Geometry: final body of the model. Coordinates: model frame, mm. Face numbers are marked on the shaded views. Give positions to 0.01 mm unless a question says otherwise; leave off trailing zeros. Loops run counter-clockwise (first coordinate to the right, second up) from the corner with the lowest first, then second, coordinate; pieces in that order, holes last. Notation, with made-up numbers: (10, 40) - (27, 40) arc R23 cw to (27, 76) - close; hole circle Ø9 at (63, 48.25). An arc over 180 degrees is marked (long way). Use one line per item in the form item = value.
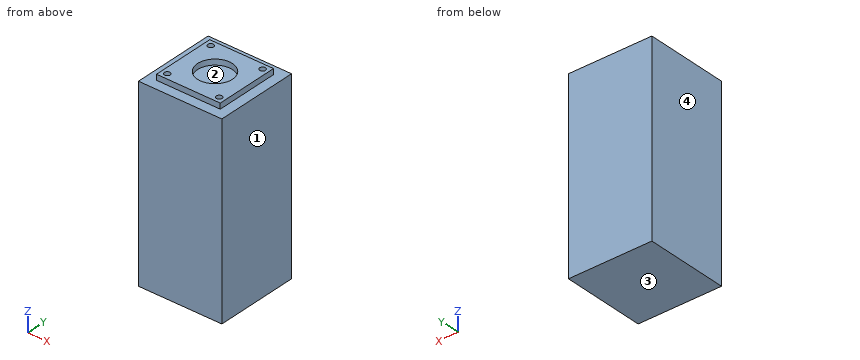
Autodesk Inventor part; units mm, degrees
ref_plane "YZ Plane" through (0, 0, 0) normal (1, 0, 0) x (0, 1, 0)
ref_plane "XZ Plane" through (0, 0, 0) normal (0, 1, 0) x (-1, 0, 0)
ref_plane "XY Plane" through (0, 0, 0) normal (0, 0, 1) x (1, 0, 0)
sketch "Sketch1" plane through (0, 0, 0) normal (0, 0, 1) x (1, 0, 0)
  line L0 (-11.25, 11.25) -> (11.25, 11.25)
  line L1 (11.25, 11.25) -> (11.25, -11.25)
  line L2 (11.25, -11.25) -> (-11.25, -11.25)
  line L3 (-11.25, -11.25) -> (-11.25, 11.25)
  line L4 (-11.25, 11.25) -> (11.25, -11.25) construction
  line L5 (11.25, 11.25) -> (-11.25, -11.25) construction
  point P0 (0, 0)
  dimension "d0" = 22.5
  dimension "d1" = 22.5
extrude "Extrusion1" add sketch "Sketch1" along normal mid plane 50.5
sketch "Sketch8" plane through (0, 0, 25.25) normal (0, 0, 1) x (1, 0, 0)
  line L0 (-8.6, 8.6) -> (8.6, 8.6)
  line L1 (8.6, 8.6) -> (8.6, -8.6)
  line L2 (8.6, -8.6) -> (-8.6, -8.6)
  line L3 (-8.6, -8.6) -> (-8.6, 8.6)
  line L4 (-8.6, 8.6) -> (8.6, -8.6) construction
  line L5 (8.6, 8.6) -> (-8.6, -8.6) construction
  circle A0 centre (0, 0) radius 4.715
  dimension "d41" = 17.2
  dimension "d42" = 17.2
  dimension "d43" = 9.43
extrude "Extrusion4" add sketch "Sketch8" along normal blind 1.5
sketch "Sketch9" plane through (0, 0, 26.75) normal (0, 0, 1) x (1, 0, 0)
  line L0 (-8.6, -8.6) -> (8.6, -8.6)
  line L1 (8.6, -8.6) -> (8.6, 8.6)
  line L2 (8.6, 8.6) -> (-8.6, 8.6)
  line L3 (-8.6, 8.6) -> (-8.6, -8.6)
  circle A0 centre (0, 0) radius 4.715
  line L4 (-8.6, -8.6) -> (8.6, -8.6)
  line L5 (8.6, -8.6) -> (8.6, 8.6)
  line L6 (8.6, 8.6) -> (-8.6, 8.6)
  line L7 (-8.6, 8.6) -> (-8.6, -8.6)
  circle A1 centre (0, 0) radius 4.715
  point P0 (-7, 7)
  point P1 (7, 7)
  point P2 (-7, -7)
  point P3 (7, -7)
  dimension "d48" = 14
  dimension "d51" = 14
  dimension "d54" = 7
  dimension "d55" = 7
hole "Hole3" at (-7, 7, 26.75) at (7, 7, 26.75) at (-7, -7, 26.75) at (7, -7, 26.75) direction (0, 0, -1) diameter 1.567 depth 3 tip angle 118
equation "\"d42\" = d41"
properties part number "toppmt"
(1) Cut plane A-A (x = 0). Return the cut outline in (y, z) (3 decimals), plus the area to 3 significant figures.
Solution:
outline = (-11.25, -25.25) - (11.25, -25.25) - (11.25, 25.25) - (8.6, 25.25) - (8.6, 26.75) - (4.715, 26.75) - (4.715, 25.25) - (-4.715, 25.25) - (-4.715, 26.75) - (-8.6, 26.75) - (-8.6, 25.25) - (-11.25, 25.25) - close
area = 1,150 mm2
(2) Cut plane B-B (x = 3.25). Return the cut outline in (y, z).
Solution:
outline = (-11.25, -25.25) - (11.25, -25.25) - (11.25, 25.25) - (8.6, 25.25) - (8.6, 26.75) - (3.42, 26.75) - (3.42, 25.25) - (-3.42, 25.25) - (-3.42, 26.75) - (-8.6, 26.75) - (-8.6, 25.25) - (-11.25, 25.25) - close
(3) Pull-direction query (X, two-part tool) for the marked faces 1, 2, 3 and 4; classes: released by +X, released by -X, zero draft, split by the parting line, or undercut.
Solution:
face_1 = released by +X
face_2 = undercut
face_3 = zero draft
face_4 = released by -X
(4) Pin query (flat end, axial travel): P1, Ø1.3, axis at x = -7, y = 7, coming from the +Z side; P2, Ø0.8, axis at y = 4, z = 26, coming from the +X side; P3, Ø1.2, axis at x = -3.5, z = 26, coming from the +Y side. Return the tip coordinate at first contact, or that it passes through.
Solution:
P1 = 23.67
P2 = 8.6
P3 = 8.6
(5) Material intervals for L1, parallel to X at y = -7, z = 25.7; L2, parallel to Y at x = -7, z = 25, sorted ascending. Write a range as from..to.
Solution:
L1 = -8.6..-7.78, -6.22..6.22, 7.78..8.6
L2 = -11.25..-7.78, -6.22..6.22, 7.78..11.25
